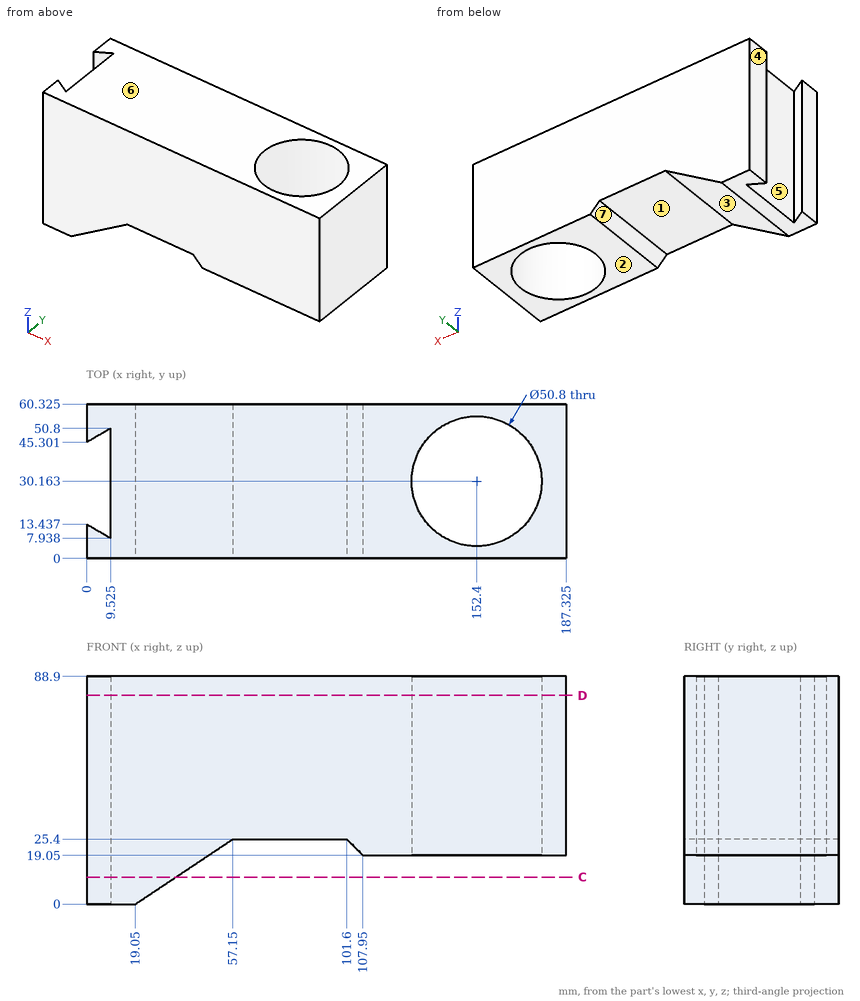
Geometry check sheet. Reference: drawing and pictorial views, mm from the part's lowest x, y, z. A direction names the side the tool comes from. Coordinates: 2 decimals unless noted, no trailing zeros. Order: outer loops, then holes, each group sorted by start corner. A loop starts at its lowest first (then second) coordinate and runs counter-clockwise, first axis right, second up. Notation, with made-up numbers: M -21.75,10.5 L -3.75,10.5 A9 ccw -3.75,26.5 Z; hole C 41.25,-21 d4. An arc over 180 degrees is marked long. Return JSON: item names as keys, results as strings.
1) Release check for a two-part mould opening along X. For the marked faces 1, 2, 3 and 4 record: +X half, -X half, draft (parallel to the pull), parting line (faces both ways), or undercut.
Answer list:
{"face 1": "undercut", "face 2": "draft", "face 3": "undercut", "face 4": "-X half"}
2) Cross-section at D-D, the plane z = 81.5. Record the boundary of the cut face in (x, y) (1 decimal), and give its area (3 significant figures).
Answer list:
{"outline": "M 0,0 L 187.3,0 L 187.3,60.3 L 0,60.3 L 0,45.3 L 9.5,50.8 L 9.5,7.9 L 0,13.4 Z; hole C 152.4,30.2 d50.8", "area": "8,920 mm2"}
3) Thickness scan on L1, parallel to Y at x = 152.4, z = 34.5 (1 decimal); L2, parallel to X at y = 46, z = 68 (1 decimal); L3, parallel to Z at x = 112, y = 10. Record the ranges inside material, lowest first. Write a range as [from, to].
Answer list:
{"L1": "[0, 4.8], [55.6, 60.3]", "L2": "[0, 1.2], [9.5, 132.5], [172.3, 187.3]", "L3": "[19.05, 88.9]"}
4) Cross-section at C-C, the plane z = 10.5. Record the boundary of the cut face in (x, y) (1 decimal), and give its area (3 significant figures).
Answer list:
{"outline": "M 0,0 L 34.8,0 L 34.8,60.3 L 0,60.3 L 0,45.3 L 9.5,50.8 L 9.5,7.9 L 0,13.4 Z", "area": "1,740 mm2"}
5) Gauge pin test, flat ends, axial feed: pin 1 (1.5 mm diameter, centred on x = 81, y = 23, fed in from -Z); pin 2 (6 mm diameter, centred on y = 21, z = 34, fed in from -X) (1 decimal). Record the tip position at first contact, or that the pin passes through.
Answer list:
{"pin 1": "z = 25.4", "pin 2": "x = 9.5"}
6) Access from +Z, -Z, +X, -X, +Y, -Y to the whole of each face (thin tool, end or side, straight path). Record for the marked faces 5, 6 and 7.
Answer list:
{"face 5": "+Z, -Z", "face 6": "+Z, +X, -X, +Y, -Y", "face 7": "-Z, +Y, -Y"}
